from build123d import *

# Parameters (mm, degrees)
F0_W     = 105.7758629322
F0_H     = 88.4018465877
F0_R     = 2.6924
F1_DEPTH = 2.5654
F2_DEPTH = 1.016
F3_R     = 2.6924
F4_DEPTH = 2.7051


with BuildPart() as f1:
    # F0 (on Top) → F1 (new body)
    with BuildSketch(Plane.XY):
        Rectangle(F0_W, F0_H)
        with BuildLine():
            ThreePointArc((-32.004, -29.337), (-30.1181462146, -30.1181462146), (-29.337, -32.004))
            ThreePointArc((-29.337, -32.004), (-33.8898537854, -33.8898537854), (-32.004, -29.337))
        make_face(mode=Mode.SUBTRACT)
        with Locations((0, -38.0238)):
            Circle(F0_R, mode=Mode.SUBTRACT)
        with BuildLine():
            ThreePointArc((32.004, -29.337), (33.8898537854, -30.1181462146), (34.671, -32.004))
            ThreePointArc((34.671, -32.004), (30.1181462146, -33.8898537854), (32.004, -29.337))
        make_face(mode=Mode.SUBTRACT)
        with BuildLine():
            ThreePointArc((-32.004, 29.337), (-33.8898537854, 33.8898537854), (-29.337, 32.004))
            ThreePointArc((-29.337, 32.004), (-30.1181462146, 30.1181462146), (-32.004, 29.337))
        make_face(mode=Mode.SUBTRACT)
        with BuildLine():
            Line((35.56, -24.13), (29.21, -29.21))
            Line((29.21, -29.21), (-29.21, -29.21))
            Line((-29.21, -29.21), (-35.56, -24.13))
            Line((-35.56, -24.13), (-35.56, -0.8929825082))
            ThreePointArc((-35.56, -0.8929825082), (-35.7124, 0), (-35.56, 0.8929825082))
            Line((-35.56, 0.8929825082), (-35.56, 24.13))
            Line((-35.56, 24.13), (-29.21, 29.21))
            Line((-29.21, 29.21), (0, 29.21))
            Line((0, 29.21), (29.21, 29.21))
            Line((29.21, 29.21), (35.56, 24.13))
            Line((35.56, 24.13), (35.56, 0.8929825082))
            ThreePointArc((35.56, 0.8929825082), (35.6740265409, 0.4529468843), (35.7124, 0))
            ThreePointArc((35.7124, 0), (35.6740265409, -0.4529468843), (35.56, -0.8929825082))
            Line((35.56, -0.8929825082), (35.56, -24.13))
        make_face(mode=Mode.SUBTRACT)
        with BuildLine():
            ThreePointArc((2.6924, 38.0238), (1.9038142977, 36.1199857023), (0, 35.3314))
            ThreePointArc((0, 35.3314), (-1.9038142977, 39.9276142977), (2.6924, 38.0238))
        make_face(mode=Mode.SUBTRACT)
        with BuildLine():
            ThreePointArc((32.004, 29.337), (30.1181462146, 33.8898537854), (34.671, 32.004))
            ThreePointArc((34.671, 32.004), (33.8898537854, 30.1181462146), (32.004, 29.337))
        make_face(mode=Mode.SUBTRACT)
        with BuildLine():
            Line((-35.56, -24.13), (-29.21, -29.21))
            Line((-29.21, -29.21), (-29.21, 29.21))
            Line((-29.21, 29.21), (-35.56, 24.13))
            Line((-35.56, 24.13), (-35.56, 0.8929825082))
            ThreePointArc((-35.56, 0.8929825082), (-32.5670531157, 2.6540265409), (-30.3276, 0))
            ThreePointArc((-30.3276, 0), (-32.5670531157, -2.6540265409), (-35.56, -0.8929825082))
            Line((-35.56, -0.8929825082), (-35.56, -24.13))
        make_face()
        with BuildLine():
            Line((29.21, 29.21), (29.21, -29.21))
            Line((29.21, -29.21), (35.56, -24.13))
            Line((35.56, -24.13), (35.56, -0.8929825082))
            ThreePointArc((35.56, -0.8929825082), (30.3276, 0), (35.56, 0.8929825082))
            Line((35.56, 0.8929825082), (35.56, 24.13))
            Line((35.56, 24.13), (29.21, 29.21))
        make_face()
        with BuildLine():
            ThreePointArc((2.6924, 38.0238), (-1.9038142977, 39.9276142977), (0, 35.3314))
            ThreePointArc((0, 35.3314), (1.9038142977, 36.1199857023), (2.6924, 38.0238))
        make_face()
        with Locations((0, -38.0238)):
            Circle(F0_R)
        with BuildLine():
            Line((-35.56, 0.8929825082), (-35.56, -0.8929825082))
            ThreePointArc((-35.56, -0.8929825082), (-32.5670531157, -2.6540265409), (-30.3276, 0))
            ThreePointArc((-30.3276, 0), (-32.5670531157, 2.6540265409), (-35.56, 0.8929825082))
        make_face()
        with BuildLine():
            ThreePointArc((35.56, 0.8929825082), (30.3276, 0), (35.56, -0.8929825082))
            Line((35.56, -0.8929825082), (35.56, 0.8929825082))
        make_face()
        with BuildLine():
            Line((35.56, 0.8929825082), (35.56, -0.8929825082))
            ThreePointArc((35.56, -0.8929825082), (35.6740265409, -0.4529468843), (35.7124, 0))
            ThreePointArc((35.7124, 0), (35.6740265409, 0.4529468843), (35.56, 0.8929825082))
        make_face()
        with BuildLine():
            ThreePointArc((-35.56, 0.8929825082), (-35.7124, 0), (-35.56, -0.8929825082))
            Line((-35.56, -0.8929825082), (-35.56, 0.8929825082))
        make_face()
    extrude(amount=F1_DEPTH)

    # F0 (on Top) → F2 (cut)
    with BuildSketch(Plane.XY):
        with BuildLine():
            Line((29.21, 29.21), (29.21, -29.21))
            Line((29.21, -29.21), (35.56, -24.13))
            Line((35.56, -24.13), (35.56, -0.8929825082))
            ThreePointArc((35.56, -0.8929825082), (30.3276, 0), (35.56, 0.8929825082))
            Line((35.56, 0.8929825082), (35.56, 24.13))
            Line((35.56, 24.13), (29.21, 29.21))
        make_face()
        with BuildLine():
            ThreePointArc((35.56, 0.8929825082), (30.3276, 0), (35.56, -0.8929825082))
            Line((35.56, -0.8929825082), (35.56, 0.8929825082))
        make_face()
        with BuildLine():
            Line((-35.56, -24.13), (-29.21, -29.21))
            Line((-29.21, -29.21), (-29.21, 29.21))
            Line((-29.21, 29.21), (-35.56, 24.13))
            Line((-35.56, 24.13), (-35.56, 0.8929825082))
            ThreePointArc((-35.56, 0.8929825082), (-32.5670531157, 2.6540265409), (-30.3276, 0))
            ThreePointArc((-30.3276, 0), (-32.5670531157, -2.6540265409), (-35.56, -0.8929825082))
            Line((-35.56, -0.8929825082), (-35.56, -24.13))
        make_face()
        with BuildLine():
            Line((-35.56, 0.8929825082), (-35.56, -0.8929825082))
            ThreePointArc((-35.56, -0.8929825082), (-32.5670531157, -2.6540265409), (-30.3276, 0))
            ThreePointArc((-30.3276, 0), (-32.5670531157, 2.6540265409), (-35.56, 0.8929825082))
        make_face()
    extrude(amount=F2_DEPTH, mode=Mode.SUBTRACT)

    # F3 (on face) → F4 (join)
    with BuildSketch(Plane.XY.offset(2.5654)):
        with Locations((0, 38.0238)):
            Circle(F3_R)
        with Locations((0, -38.0238)):
            Circle(F3_R)
        with Locations((33.02, 0)):
            Circle(F3_R)
        with Locations((-33.02, 0)):
            Circle(F3_R)
    extrude(amount=F4_DEPTH)


solid = f1.part
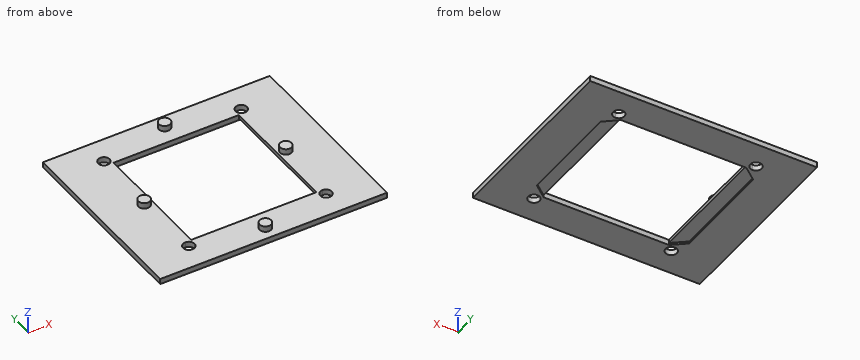
Here's how the part is built. I have some questions about the finished solid (model axes, mm). Coordinates: 2 decimals unless noted, no trailing zeros. Write each loop counter-clockwise with the first axis right and the second up, starting at its lowest first coordinate (ties: lowest second). Pieces come first, ordered by that corner, then holes.
1) If we section it at C-C (y = -17): List the corners of the cut face in (x, z) for me, plus the area to 3 significant figures.
Filled in:
outline: (-52.89, 0) - (-35.56, 0) - (-35.56, 1.02) - (-29.21, 1.02) - (-29.21, 2.57) - (-52.89, 2.57) - close; (29.21, 1.02) - (35.56, 1.02) - (35.56, 0) - (52.89, 0) - (52.89, 2.57) - (29.21, 2.57) - close
area: 109 mm2
2) I'm going to push flat-ended pins straight in: pin 1 (3 mm diameter, centred on x = 32.004, y = 32.004, fed in from +Z); pin 2 (1.9 mm diameter, centred on x = 32.5, y = -2.5, fed in from -Z); pin 3 (7 mm diameter, centred on x = -32.004, y = 32.004, fed in from +Z). Where does each tip first touch, or does it pass through?
Filled in:
pin 1: passes through
pin 2: stops at z = 1.02
pin 3: stops at z = 2.57
3) If we section it at D-D (z = 3.8): List the corners of the cut face in (x, y) for me, plus the area to 3 significant figures.
Filled in:
outline: circle Ø5.38 at (-33.02, 0); circle Ø5.38 at (0, -38.02); circle Ø5.38 at (0, 38.02); circle Ø5.38 at (33.02, 0)
area: 91.1 mm2
4) If we section it at A-A (y = 0): List the corners of the cut face in (x, z) for me.
Filled in:
outline: (-52.89, 0) - (-35.56, 0) - (-35.56, 1.02) - (-29.21, 1.02) - (-29.21, 2.57) - (-30.33, 2.57) - (-30.33, 5.27) - (-35.71, 5.27) - (-35.71, 2.57) - (-52.89, 2.57) - close; (29.21, 1.02) - (35.56, 1.02) - (35.56, 0) - (52.89, 0) - (52.89, 2.57) - (35.71, 2.57) - (35.71, 5.27) - (30.33, 5.27) - (30.33, 2.57) - (29.21, 2.57) - close
5) If we section it at B-B (x = 17): List the corners of the cut face in (y, z) for me.
Filled in:
outline: (-44.2, 0) - (-29.21, 0) - (-29.21, 2.57) - (-44.2, 2.57) - close; (29.21, 0) - (44.2, 0) - (44.2, 2.57) - (29.21, 2.57) - close
6) If I drill on line 1 (X direction, y = -29, z = 2.45); line 2 (X direction, y = 12, z = 0.4); line 3 (Y direction, x = -20, z = 0.9), over which ranges is the centre line in solid material (lowest first)?
Filled in:
line 1: x = -52.89 to -29.21, 29.21 to 52.89
line 2: x = -52.89 to -35.56, 35.56 to 52.89
line 3: y = -44.2 to -29.21, 29.21 to 44.2
